Can you work these out from the model? Positions are in its coordinate system, mm. Face numbers are marked on the shaded views. A direction names the side the tool comes from. Give positions to 0.01 mm unless a question says otherwise; leave off trailing zeros. Loops run counter-clockwise (first coordinate to the right, second up) from the corner with the lowest first, then second, coordinate; pieces in that order, holes last.
from build123d import *

# Parameters (mm, degrees)
SKETCH1_W               = 8
SKETCH1_H               = 8
BOSS_EXTRUDE1_DEPTH     = 3
CUT_EXTRUDE1_DEPTH      = 12.704699911
CUT_EXTRUDE1_DEPTH_BACK = 12.704699911
CUT_EXTRUDE2_DEPTH      = 11
SKETCH4_R               = 1.8
CUT_EXTRUDE3_DEPTH      = 0.8
SKETCH5_W               = 8
SKETCH5_H               = 1
BOSS_EXTRUDE2_DEPTH     = 2
FILLET1_R               = 4
CUT_EXTRUDE4_DEPTH      = 0.4


with BuildPart() as part:
    # Sketch1 → Boss-Extrude1 (new body)
    with BuildSketch(Plane(origin=(0, 0, 0), x_dir=(1, 0, 0), z_dir=(0, 1, 0))):
        with Locations((4, 4)):
            Rectangle(SKETCH1_W, SKETCH1_H)
    extrude(amount=BOSS_EXTRUDE1_DEPTH)

    # Sketch2 → Cut-Extrude1 (cut, two sides: drawn at the far end of the back side and taken through both)
    with BuildSketch(Plane.XY.offset(-CUT_EXTRUDE1_DEPTH_BACK)):
        Polygon((0, 0), (0.6, 3), (0, 3), align=None)
        Polygon((8, 0), (7.4, 3), (8, 3), align=None)
    extrude(amount=CUT_EXTRUDE1_DEPTH + CUT_EXTRUDE1_DEPTH_BACK, mode=Mode.SUBTRACT)

    # Sketch3 → Cut-Extrude2 (cut)
    with BuildSketch(Plane(origin=(0, 0, 0), x_dir=(0, 0, -1), z_dir=(1, 0, 0))):
        Polygon((0, 0), (0.6, 3), (0, 3), align=None)
        Polygon((8, 3), (7.4, 3), (8, 0), align=None)
    extrude(amount=CUT_EXTRUDE2_DEPTH, mode=Mode.SUBTRACT)

    # Sketch4 → Cut-Extrude3 (cut)
    with BuildSketch(Plane.XZ):
        with Locations(Location((4, -3.75, 0), (0, 0, 270))):
            Circle(SKETCH4_R)
    extrude(amount=-CUT_EXTRUDE3_DEPTH, mode=Mode.SUBTRACT)

    # Sketch5 → Boss-Extrude2 (add)
    with BuildSketch(Plane.XZ):
        with Locations((4, -7.5)):
            Rectangle(SKETCH5_W, SKETCH5_H)
    extrude(amount=BOSS_EXTRUDE2_DEPTH)

    # Fillet1
    # the kernel refuses this fillet: 4 mm, written as the material it takes off along each edge
    with BuildSketch(Plane(origin=(8, -2, -16.660254038), x_dir=(0, 1, 0), z_dir=(0, 0, 1)), Plane(origin=(0, -2, 1.660254038), x_dir=(0, 1, 0), z_dir=(0, 0, -1))) as fillet1_piece_1:
        with BuildLine():
            CenterArc((4, 3.464101615), FILLET1_R, 180, 60)
            Line((0, 3.464101615), (-0.08, 3.464101615))
            Line((-0.08, 3.464101615), (-0.08, 0))
            Line((-0.08, 0), (0, -0.08))
            ThreePointArc((0, -0.08), (1, -0.08), (1.96, -0.069282032))
            Line((1.96, -0.069282032), (2, 0))
        make_face()
    extrude(amount=18.320508076, mode=Mode.SUBTRACT)

    # Sketch6 → Cut-Extrude4 (cut)
    with BuildSketch(Plane(origin=(0, 3, 0), x_dir=(1, 0, 0), z_dir=(0, 1, 0))):
        with BuildLine():
            Line((3.443331895, 5.130686034), (4.597178049, 5.130686034))
            Line((4.597178049, 5.130686034), (4.597178049, 4.291743727))
            add(Edge.make_bspline(
                [(4.597178049, 4.291743727), (4.596645702, 4.211170655), (4.595640561, 4.059038126), (4.578021597, 3.844434295), (4.553540207, 3.655975372), (4.51459395, 3.491238943), (4.462448704, 3.342468302), (4.388723742, 3.206338125), (4.298056147, 3.076066307), (4.187154731, 2.955594738), (4.059577941, 2.844170634), (3.913847481, 2.747275335), (3.753421756, 2.660946408), (3.638168327, 2.615497851), (3.579149203, 2.592224496)],
                knots=[0, 0, 0, 0, 1.347156832, 2.543608823, 3.599300285, 4.522475688, 5.370350604, 6.227678973, 7.103274953, 8.018757603, 8.959280198, 9.929437417, 10.939703653, 12, 12, 12, 12], degree=3))
            Line((3.579149203, 2.592224496), (3.366408818, 3.053762957))
            add(Edge.make_bspline(
                [(3.366408818, 3.053762957), (3.417874874, 3.07492834), (3.516080495, 3.11531534), (3.647721841, 3.193115232), (3.754216523, 3.284666717), (3.839841548, 3.388423011), (3.901059293, 3.510472084), (3.947065575, 3.648752862), (3.973734578, 3.806802537), (3.979016553, 3.918249261), (3.981793434, 3.976839881)],
                knots=[0, 0, 0, 0, 1.113959817, 2.125616841, 3.047494432, 3.914868512, 4.801521967, 5.765947312, 6.825496818, 8, 8, 8, 8], degree=3))
            Line((3.981793434, 3.976839881), (3.443331895, 3.976839881))
            Line((3.443331895, 3.976839881), (3.443331895, 5.130686034))
        make_face()
    extrude(amount=-CUT_EXTRUDE4_DEPTH, mode=Mode.SUBTRACT)


solid = part.part
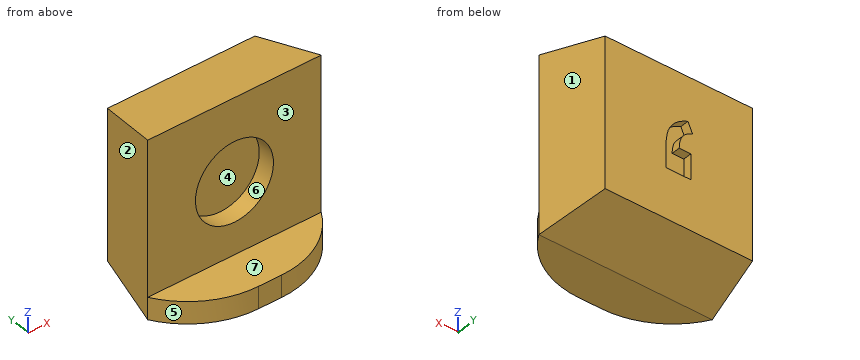
(1) Suppose I cut it at B-B on x = 3. List the corners of the cut face in (y, z) for me.
Returned:
outline: (-1.97, -8) - (0, -8) - (3, -7.4) - (3, -0.6) - (0, 0) - (0, -2.25) - (0.8, -2.25) - (0.8, -5.25) - (0, -5.25) - (0, -7) - (-1.97, -7) - close
(2) Suppose I cut it at C-C on y = 2.2. List the corners of the cut face in (x, z) for me, plus the area to 3 significant figures.
Returned:
outline: (0.44, -7.56) - (7.56, -7.56) - (7.56, -0.44) - (0.44, -0.44) - close
area: 50.7 mm2
(3) Which directions (+Z, -Z, +X, -X, +Y, -Y) give clear straight access to the entire face, cutting with the end or side of a thin tool? Please do the marked faces 5, 6 and 7.
Returned:
face 5: +Z, -Z, -X, -Y
face 6: -Y
face 7: +Z, +X, -X, -Y
(4) Suppose I cut it at A-A on z = -7.5. List the corners of the cut face in (x, y) for me, plus the area to 3 significant figures.
Returned:
outline: (0, 0) arc R4 ccw to (3.46, -2) - (4.54, -2) arc R4 ccw to (8, 0) - (7.5, 2.5) - (0.5, 2.5) - close
area: 30.7 mm2
(5) Will these pins go through, and if not, where does the flat tip stop? P1, Ø1, axis at y = 2, z = -6.5, coming from the -X side; P2, Ø1.1, axis at x = 4, z = -3, coming from the -Y side; P3, Ø1, axis at y = 1, z = -1.5, coming from the +X side.
Returned:
P1: stops at x = 0.3
P2: stops at y = 0.8
P3: stops at x = 7.9
(6) Suppose I cut it at D-D on z = -6. List the corners of the cut face in (x, y) for me, plus the area to 3 significant figures.
Returned:
outline: (0, 0) - (8, 0) - (7.4, 3) - (0.6, 3) - close
area: 22.2 mm2
(7) Please list where these lines run through material, in increasing order: probe 1 along Y at (x, z) = (5, -1.5); probe 2 along Z at (x, y) = (1, -0.5); probe 3 along Y at (x, z) = (2.75, -4).
Returned:
probe 1: y = 0 to 3
probe 2: z = -8 to -7
probe 3: y = 0.8 to 3
(8) Thinking about a two-plate mould opening in X: for the marked faces 1, 2, 3 and 4, which applies, pulls with the +X half, pulls with the -X half, needs draft (parallel to the pull), parting line crosses it, or undercut?
Returned:
face 1: pulls with the +X half
face 2: pulls with the -X half
face 3: needs draft
face 4: undercut
